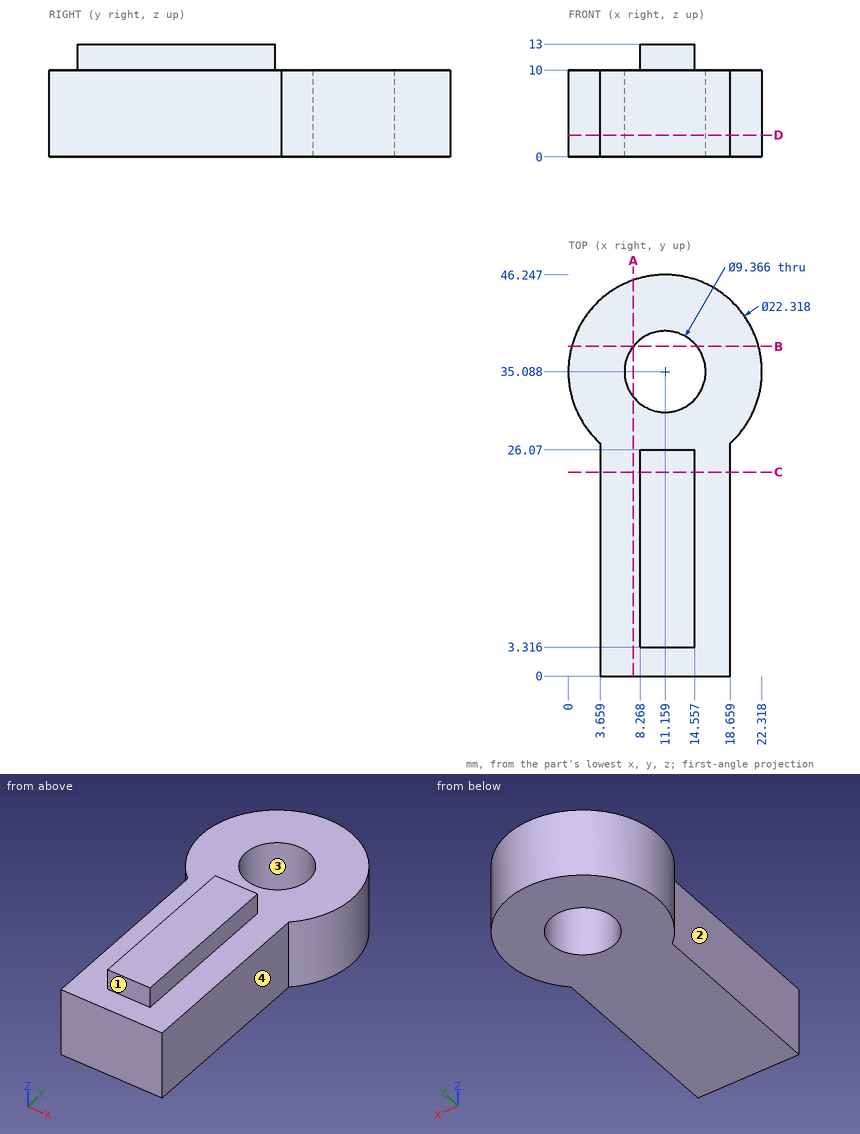
Input: dimensioned drawing with shaded views. Units: mm. Origin: part minimum x, y, z. Give positions to 0.01 mm unless a question says otherwise; leave off trailing zeros. Loops run counter-clockwise (first coordinate to the right, second up) from the corner with the lowest first, then second, coordinate; pieces in that order, holes last. Notation, with made-up numbers: (69.25, -15.5) -> (116.25, -15.5) arc R27 ccw to (116.25, 14.5) -> close; hole circle Ø8 at (77, -22). An arc over 180 degrees is marked (long way). Use a Markdown table: item, result.
Q1. Section query A-A, the plane x = 7.5. Return the cut outline in (y, z) (1 decimal), plus the area to 3 significant figures.
Entries:
| item | result |
|---|---|
| outline | (0, 0) -> (32.2, 0) -> (32.2, 10) -> (0, 10) -> close; (38, 0) -> (45.6, 0) -> (45.6, 10) -> (38, 10) -> close |
| area | 398 mm² |
Q2. Section query C-C, the plane y = 23.5. Return the cut outline in (x, z).
Entries:
| item | result |
|---|---|
| outline | (3.66, 0) -> (18.66, 0) -> (18.66, 10) -> (14.56, 10) -> (14.56, 13) -> (8.27, 13) -> (8.27, 10) -> (3.66, 10) -> close |
Q3. Section query B-B, the plane y = 38. Return the cut outline in (x, z), plus the area to 3 significant figures.
Entries:
| item | result |
|---|---|
| outline | (0.39, 0) -> (7.49, 0) -> (7.49, 10) -> (0.39, 10) -> close; (14.83, 0) -> (21.93, 0) -> (21.93, 10) -> (14.83, 10) -> close |
| area | 142 mm² |
Q4. Ray query, probe 1 along X at (y, z) = (11, 6); probe 2 along X at (y, z) = (9, 11.75); probe 3 along Z at (x, y) = (4, 35). Return the intervals inside material, ascending. Write a range as from..to.
Entries:
| item | result |
|---|---|
| probe 1 | x = 3.66..18.66 |
| probe 2 | x = 8.27..14.56 |
| probe 3 | z = 0..10 |
Q5. Section query D-D, the plane z = 2.5. Return the cut outline in (x, y) (1 decimal).
Entries:
| item | result |
|---|---|
| outline | (3.7, 0) -> (18.7, 0) -> (18.7, 26.8) arc R11.2 ccw (long way) to (3.7, 26.8) -> close; hole circle Ø9.4 at (11.2, 35.1) |
Q6. First-contact query: P1, Ø0.9, axis at y = 18, z = 11, coming from the +X side; P2, Ø3.5, axis at y = 13, z = 11, coming from the -X side; P3, Ø0.9, axis at x = 12, z = 11, coming from the +Y side. Flat tips, straight axial feed; report the tip coordinate or a pass-through.
Entries:
| item | result |
|---|---|
| P1 | stops at x = 14.56 |
| P2 | stops at x = 3.66 |
| P3 | stops at y = 26.07 |
Q7. Pull-direction query (X, two-part tool) for the marked faces 1, 2, 3 and 4; classes: pulls with the +X half, pulls with the -X half, needs draft (parallel to the pull), parting line crosses it, or undercut.
Entries:
| item | result |
|---|---|
| face 1 | needs draft |
| face 2 | pulls with the -X half |
| face 3 | undercut |
| face 4 | pulls with the +X half |
